Build history of the part. All positions in model axes, mm. A direction names the side the tool comes from. Give positions to 0.01 mm unless a question says otherwise; leave off trailing zeros. Order: outer loops, then holes, each group sorted by start corner. A loop starts at its lowest first (then second) coordinate and runs counter-clockwise, first axis right, second up. Notation, with made-up numbers: (-25, 29) - (-3, 29) arc R5 cw to (-3, 37) - close; hole circle Ø2 at (-23, 67.5). An arc over 180 degrees is marked (long way). One line per item, written item: value.
```python
from build123d import *

# Parameters (mm, degrees)
SKETCH1_R           = 1.7
BOSS_EXTRUDE1_DEPTH = 38
CUT_EXTRUDE1_DEPTH  = 38
SKETCH3_R           = 1.7
CUT_EXTRUDE2_DEPTH  = 9


with BuildPart() as part:
    # Sketch1 → Boss-Extrude1 (new body)
    with BuildSketch(Plane.XY):
        Polygon((-194.023766161, 235.92362241), (-230.573766163, 235.92362241), (-230.573766163, 210.92362241), (-194.023766161, 210.92362241), (-194.023766161, 223.42362241), align=None)
        with Locations((-225.573766163, 216.92362241)):
            Circle(SKETCH1_R, mode=Mode.SUBTRACT)
        with Locations((-225.573766163, 229.92362241)):
            Circle(SKETCH1_R, mode=Mode.SUBTRACT)
    extrude(amount=BOSS_EXTRUDE1_DEPTH)

    # Sketch2 → Cut-Extrude1 (cut)
    with BuildSketch(Plane(origin=(0, 235.92362241, 0), x_dir=(1, 0, 0), z_dir=(0, 1, 0))):
        with BuildLine():
            Line((-213.078407846, 0), (-213.078407846, -16.742061243))
            ThreePointArc((-213.078407846, -16.742061243), (-210.979515598, -32.649316271), (-211.078407846, -16.604493694))
            Line((-211.078407846, -16.604493694), (-211.078407846, 0))
            Line((-211.078407846, 0), (-213.078407846, 0))
        make_face()
        with BuildLine():
            ThreePointArc((-199.916412956, -21.613593286), (-212.016456661, -36.620181105), (-222.864018355, -20.684713088))
            Line((-222.864018355, -20.684713088), (-219.873766163, -3))
            Line((-219.873766163, -3), (-230.573766163, -3))
            Line((-230.573766163, -3), (-230.573766163, -38))
            Line((-230.573766163, -38), (-194.023766161, -38))
            Line((-194.023766161, -38), (-194.023766161, -3))
            Line((-194.023766161, -3), (-204.750473292, -3))
            Line((-204.750473292, -3), (-199.916412956, -21.613593286))
        make_face()
    extrude(amount=-CUT_EXTRUDE1_DEPTH, mode=Mode.SUBTRACT)

    # Sketch3 → Cut-Extrude2 (cut)
    with BuildSketch(Plane(origin=(0, 0, 0), x_dir=(-1, 0, 0), z_dir=(0, 0, -1))):
        with Locations((199.050473293, 216.92362241)):
            Circle(SKETCH3_R)
        with Locations((199.050473293, 229.92362241)):
            Circle(SKETCH3_R)
    extrude(amount=-CUT_EXTRUDE2_DEPTH, mode=Mode.SUBTRACT)


solid = part.part
```
(1) Slice it at B-B, the plane y = 214.75. Give the cut face in (x, z), and give its area (3 significant figures).
Completed:
outline: (-230.57, 0) - (-213.08, 0) - (-213.08, 16.74) arc R8.04 cw (long way) to (-211.08, 16.6) - (-211.08, 0) - (-194.02, 0) - (-194.02, 3) - (-204.75, 3) - (-199.92, 21.61) arc R12 ccw (long way) to (-222.86, 20.68) - (-219.87, 3) - (-230.57, 3) - close
area: 527 mm²
(2) 3-axis set-ups, long thin cutter, end or side, ignore diameter. For faces 1 (the face through (-213.078, 224, 8)), 2 (the face through (-225, 224, 3)), 3 (the face through (-199.8, 215.4, 1.5)): which of +Z, -Z, +X, -X, +Y, -Y reach the whole face in a straight line?
Completed:
face 1: -Z, +Y, -Y
face 2: -X, +Y, -Y
face 3: -Z
(3) Pin check, flat tips, straight feed: P1, Ø12, axis at y = 225, z = 15, coming from the -X side; P2, Ø5.5, axis at x = -199.05, y = 229.92, coming from the +Z side; P3, Ø3, axis at x = -200.5, y = 221, coming from the +Z side. Stop position of each tip, or through.
Completed:
P1: x = -222.97
P2: z = 31.65
P3: z = 31.92
(4) Slice it at C-C, the plane x = -220.5. Give the cut face in (y, z).
Completed:
outline: (210.92, 0) - (235.92, 0) - (235.92, 3) - (210.92, 3) - close; (210.92, 6.7) - (235.92, 6.7) - (235.92, 32.6) - (210.92, 32.6) - close
(5) Pull direction X, two halves, no side cores. Call faces 4 (the face through (-211.078, 224, 8)), 5 (the face through (-194.024, 223, 1)), 6 (the face through (-203, 224, 0)): +X half, -X half, draft (parallel to the pull), parting line (faces both ways), or undercut.
Completed:
face 4: undercut
face 5: +X half
face 6: draft
(6) Slice it at D-D, the plane x = -225. Give the cut face in (y, z), and give its area (3 significant figures).
Completed:
outline: (210.92, 0) - (215.32, 0) - (215.32, 3) - (210.92, 3) - close; (218.52, 0) - (228.32, 0) - (228.32, 3) - (218.52, 3) - close; (231.52, 0) - (235.92, 0) - (235.92, 3) - (231.52, 3) - close
area: 55.8 mm²
(7) Drill centre lines: line 1 (X direction, y = 229.75, z = 24.63); line 2 (X direction, y = 223.5, z = 14); line 3 (Z direction, x = -227.5, y = 230.75). Where is each one in solid material? Low to high.
Completed:
line 1: -223.53 to -219.57, -203.49 to -199.53
line 2: -221.73 to -213.08, -211.08 to -201.89
line 3: 0 to 3
(8) Slice it at A-A, the plane z = 24.63. Give the cut face in (x, y), and give its area (3 significant figures).
Completed:
outline: (-223.53, 210.92) - (-219.57, 210.92) - (-219.57, 235.92) - (-223.53, 235.92) - close; (-203.49, 210.92) - (-199.53, 210.92) - (-199.53, 235.92) - (-203.49, 235.92) - close
area: 198 mm²
